Verification items for the finished model (mm, model axes). Face numbers are marked on the shaded views. A direction names the side the tool comes from. Give positions to 0.01 mm unless a question says otherwise; leave off trailing zeros. Write each loop counter-clockwise with the first axis right and the second up, starting at its lowest first coordinate (ties: lowest second). Pieces come first, ordered by that corner, then holes. Notation, with made-up numbers: (42, 34.5) - (88, 34.5) arc R9 ccw to (88, 46.5) - close; hole circle Ø6 at (20, 83). An arc over 180 degrees is marked (long way). Answer as a JSON object with one key per item and string values. Group by question number.
Item 1: Sectioned sample at B-B, the plane y = -13. Record the boundary of the cut face in (x, z).
Item 2: Draft check along X on the marked faces 4, 5 and 6. Enter one of: +X half, -X half, draft (parallel to the pull), parting line (faces both ways), or undercut.
Item 3: Scan lines: line 1 along Y through (x, z) = (1.5, 1.7); line 2 along X through (y, z) = (-9.5, 2.75); line 3 along Y through (x, z) = (-9.5, 5.5). Record each from-to range of solid material in increasing order. Write a range as [from, to].
Item 4: Tool access check on the marked faces 1, 2 and 3. Record the directions out of +Z, -Z, +X, -X, +Y, -Y that give a thin tool (end or side, any length) a straight path to the whole face; none if there is none.
Item 5: Go/stop test with flat-tipped pins: pin 1 (1 mm diameter, centred on x = -5.5, y = 5, fed in from -Z); pin 2 (4 mm diameter, centred on x = 1.5, y = 9.5, fed in from +Z); pin 3 (1 mm diameter, centred on x = 0, z = 6.5, fed in from -Y); pin 4 (2.5 mm diameter, centred on x = 2, y = 12, fed in from +Z). Record where each tip stops, or that it passes through.
Item 6: Sectioned sample at A-A, the plane y = -9.5. Record the boundary of the cut face in (x, z), and give its area (3 significant figures).
Item 7: Sectioned sample at C-C, the plane x = 8.5. Record the boundary of the cut face in (y, z), and give its area (3 significant figures).
Item 8: Sectioned sample at D-D, the plane z = 5. Record the boundary of the cut face in (x, y), and give its area (3 significant figures).
```python
from build123d import *

# Parameters (mm, degrees)
SKETCHBUTTOM_W                   = 35
SKETCHBUTTOM_H                   = 30
BOSSEXTRUDEBUTTOM_DEPTH          = 10
CUTEXTRUDEFINGERROOM_START       = 4
CUTEXTRUDEFINGERROOM_DEPTH       = 6
FILLETTOP_R                      = 2
CUTEXTRUDEFINGERSHAFT_DEPTH      = 26.124689053
CUTEXTRUDEFINGERSHAFT_DEPTH_BACK = 26.124689053
SKETCHFINGERSHAFT_R              = 0.5
CUTEXTRUDESENSORROOM_START       = 3
SKETCH12_W                       = 2
SKETCH12_H                       = 10.4
CUTEXTRUDESENSORROOM_DEPTH       = 3
FILLETSENSORROOM_R               = 1
SKETCHFIXTUREHOLES_R             = 1.75
CUTEXTRUDEFIXTUREHOLES_DEPTH     = 5


with BuildPart() as part:
    # SketchButtom → BossExtrudeButtom (new body)
    with BuildSketch(Plane.XY):
        Rectangle(SKETCHBUTTOM_W, SKETCHBUTTOM_H)
    extrude(amount=BOSSEXTRUDEBUTTOM_DEPTH)

    # SketchFingerRoom → CutExtrudeFingerRoom (cut)
    with BuildSketch(Plane.XY.offset(CUTEXTRUDEFINGERROOM_START)):
        Polygon((5, 9.024), (17.5, 9.024), (17.5, -9.024), (5, -9.024), (5, -15), (-2, -15), (-2, -9.024), (-17.5, -9.024), (-17.5, 9.024), (-2, 9.024), (-2, 15), (5, 15), align=None)
    extrude(amount=CUTEXTRUDEFINGERROOM_DEPTH, mode=Mode.SUBTRACT)

    # FilletTop
    fillettop_edges = [part.edges().sort_by_distance(p)[0] for p in [
        (17.5, -12.012, 10),
        (-17.5, -12.012, 10),
        (17.5, 12.012, 10),
        (-2, 12.012, 4),
        (-2, -12.012, 4),
        (5, -12.012, 4),
        (5, 12.012, 4),
        (-2, 12.012, 10),
        (-2, -12.012, 10),
        (5, -12.012, 10),
        (5, 12.012, 10),
        (-17.5, 12.012, 10),
    ]]
    fillet(fillettop_edges, radius=FILLETTOP_R)

    # SketchFingerShaft → CutExtrudeFingerShaft (cut, two sides: drawn at the far end of the back side and taken through both)
    with BuildSketch(Plane(origin=(0, 0, 0), x_dir=(1, 0, 0), z_dir=(0, 1, 0)).offset(-CUTEXTRUDEFINGERSHAFT_DEPTH_BACK)):
        with Locations(Location((-13.5, -7, 0), (0, 0, 270))):
            Circle(SKETCHFINGERSHAFT_R)
        with Locations(Location((13.5, -7, 0), (0, 0, 270))):
            Circle(SKETCHFINGERSHAFT_R)
    extrude(amount=CUTEXTRUDEFINGERSHAFT_DEPTH + CUTEXTRUDEFINGERSHAFT_DEPTH_BACK, mode=Mode.SUBTRACT)

    # Sketch12 → CutExtrudeSensorRoom (cut)
    with BuildSketch(Plane.XY.offset(CUTEXTRUDESENSORROOM_START)):
        with Locations((5.5, 0)):
            Rectangle(SKETCH12_W, SKETCH12_H)
    extrude(amount=CUTEXTRUDESENSORROOM_DEPTH, mode=Mode.SUBTRACT)

    # FilletSensorRoom
    filletsensorroom_edges = [part.edges().sort_by_distance(p)[0] for p in [
        (4.5, 0, 4),
        (6.5, 0, 4),
    ]]
    fillet(filletsensorroom_edges, radius=FILLETSENSORROOM_R - 0.0001)  # a hair under: the kernel refuses the full size

    # SketchFixtureHoles → CutExtrudeFixtureHoles (cut, symmetric)
    with BuildSketch(Plane.XY):
        with Locations(Location((1.5, -9.5, 0), (0, 0, 15.783313229))):
            Circle(SKETCHFIXTUREHOLES_R)
        with Locations(Location((1.5, 9.5, 0), (0, 0, 344.216686771))):
            Circle(SKETCHFIXTUREHOLES_R)
    extrude(amount=CUTEXTRUDEFIXTUREHOLES_DEPTH, both=True, mode=Mode.SUBTRACT)


solid = part.part
```
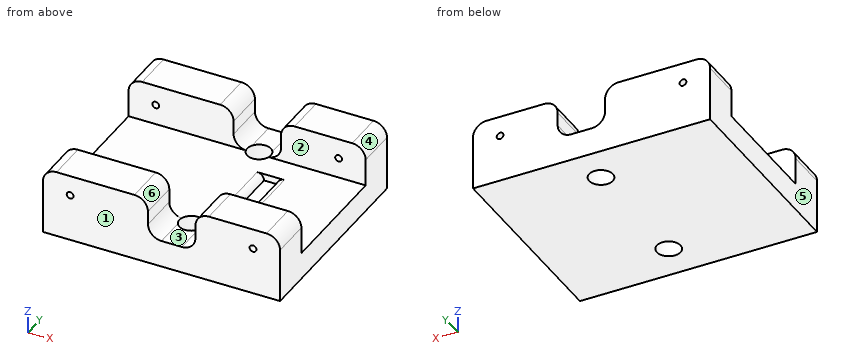
Geometry check:
{
 "1": {"outline": "(-17.5, 0) - (17.5, 0) - (17.5, 8) arc R2 ccw to (15.5, 10) - (7, 10) arc R2 ccw to (5, 8) - (5, 6) arc R2 cw to (3, 4) - (0, 4) arc R2 cw to (-2, 6) - (-2, 8) arc R2 ccw to (-4, 10) - (-15.5, 10) arc R2 ccw to (-17.5, 8) - close; hole circle Ø1 at (-13.5, 7); hole circle Ø1 at (13.5, 7)"},
 "2": {"face 4": "+X half", "face 5": "-X half", "face 6": "undercut"},
 "3": {"line 1": "[-15, -11.25], [-7.75, 7.75], [11.25, 15]", "line 2": "[-17.5, -0.25], [3.25, 17.5]", "line 3": "[-15, -9.02], [9.02, 15]"},
 "4": {"face 1": "+Z, -Z, +X, -X, -Y", "face 2": "+Z, +X, -X", "face 3": "+Z, +Y, -Y"},
 "5": {"pin 1": "z = 0", "pin 2": "z = 4.06", "pin 3": "through", "pin 4": "z = 4.02"},
 "6": {"outline": "(-17.5, 0) - (-0.25, 0) - (-0.25, 4.02) arc R2 cw to (-2, 6) - (-2, 8) arc R2 ccw to (-4, 10) - (-15.5, 10) arc R2 ccw to (-17.5, 8) - close; (3.25, 0) - (17.5, 0) - (17.5, 8) arc R2 ccw to (15.5, 10) - (7, 10) arc R2 ccw to (5, 8) - (5, 6) arc R2 cw to (3.25, 4.02) - close; hole circle Ø1 at (-13.5, 7); hole circle Ø1 at (13.5, 7)", "area": "291 mm^2"},
 "7": {"outline": "(-15, 0) - (15, 0) - (15, 10) - (9.02, 10) - (9.02, 4) - (-9.02, 4) - (-9.02, 10) - (-15, 10) - close", "area": "192 mm^2"},
 "8": {"outline": "(-17.5, -15) - (-1.73, -15) - (-1.73, -9.02) - (-17.5, -9.02) - close; (-17.5, 9.02) - (-1.73, 9.02) - (-1.73, 15) - (-17.5, 15) - close; (4.73, -15) - (17.5, -15) - (17.5, -9.02) - (4.73, -9.02) - close; (4.73, 9.02) - (17.5, 9.02) - (17.5, 15) - (4.73, 15) - close", "area": "341 mm^2"}
}
